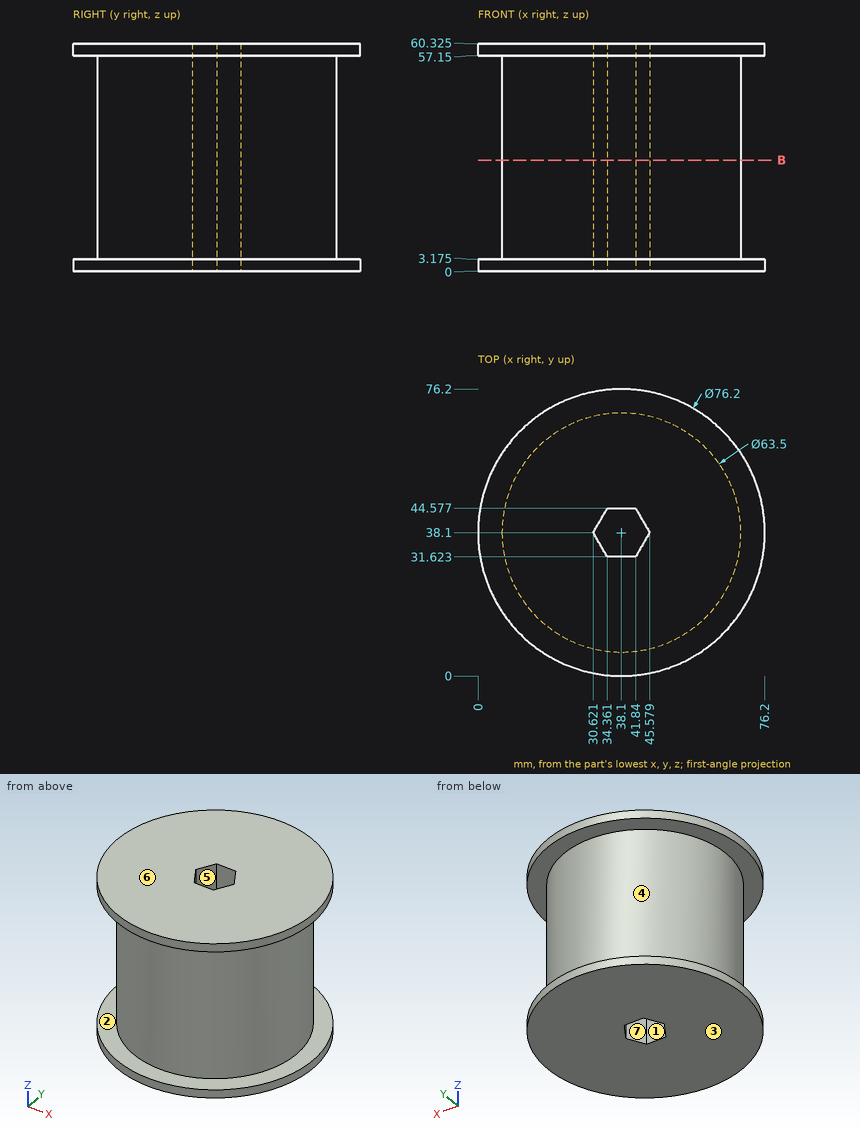
Here's the drawing with two shaded views (mm, measured from the low corner). I have some questions. A direction names the side the tool comes from. Give positions to 0.01 mm unless a question says otherwise; leave off trailing zeros. Loops run counter-clockwise (first coordinate to the right, second up) from the corner with the lowest first, then second, coordinate; pieces in that order, holes last. Notation, with made-up numbers: M 36.25,4.5 L 51.25,4.5 A24 ccw 51.25,28.5 Z; hole C -12.5,55 d6. An arc over 180 degrees is marked long. Use one line per item in the form item = value. Start each with the question number.
(1) I want a section at B-B, the plane z = 29.5. Write out the boundary of the cut face in (x, y).
(2) On a 3-axis mill with a long thin cutter (end or side, diameter ignored), from which of +Z, -Z, +X, -X, +Y, -Y can I reach the whole of each face in a straight line? I mean the marked faces 1, 2 and 3. Say none if no direction works.
(3) Thinking about a two-plate mould opening in X: for the marked faces 4, 5, 6 and 7, which applies, released by +X, released by -X, zero draft, split by the parting line, or undercut?
(4) Please list where these lines run through material, in increasing order: line 1 (Y direction, x = 39, z = 40); line 2 (X direction, y = 35.5, z = 26.5) (1 decimal); line 3 (X direction, y = 39, z = 29).
(5) I'm going to push flat-ended pins straight in: P1, Ø3.5, axis at x = 37, z = 40.5, coming from the -Y side; P2, Ø4, axis at y = 24, z = 48, coming from the +X side (1 decimal); P3, Ø3, axis at y = 18, z = 13, coming from the -X side; P4, Ø2, axis at x = 42, y = 58, coming from the -Z side. Where does each tip first touch, or does it pass through?
Worked out:
q1.outline = C 38.1,38.1 d63.5; hole M 30.62,38.1 L 34.36,31.62 L 41.84,31.62 L 45.58,38.1 L 41.84,44.58 L 34.36,44.58 Z
q2.face_1 = +Z, -Z
q2.face_2 = none
q2.face_3 = -Z, +X, -X, +Y, -Y
q3.face_4 = split by the parting line
q3.face_5 = undercut
q3.face_6 = zero draft
q3.face_7 = undercut
q4.line_1 = 6.36 to 31.62, 44.58 to 69.84
q4.line_2 = 6.5 to 32.1, 44.1 to 69.7
q4.line_3 = 6.36 to 31.14, 45.06 to 69.84
q5.P1 = 6.35
q5.P2 = 67.5
q5.P3 = 12.37
q5.P4 = 0
